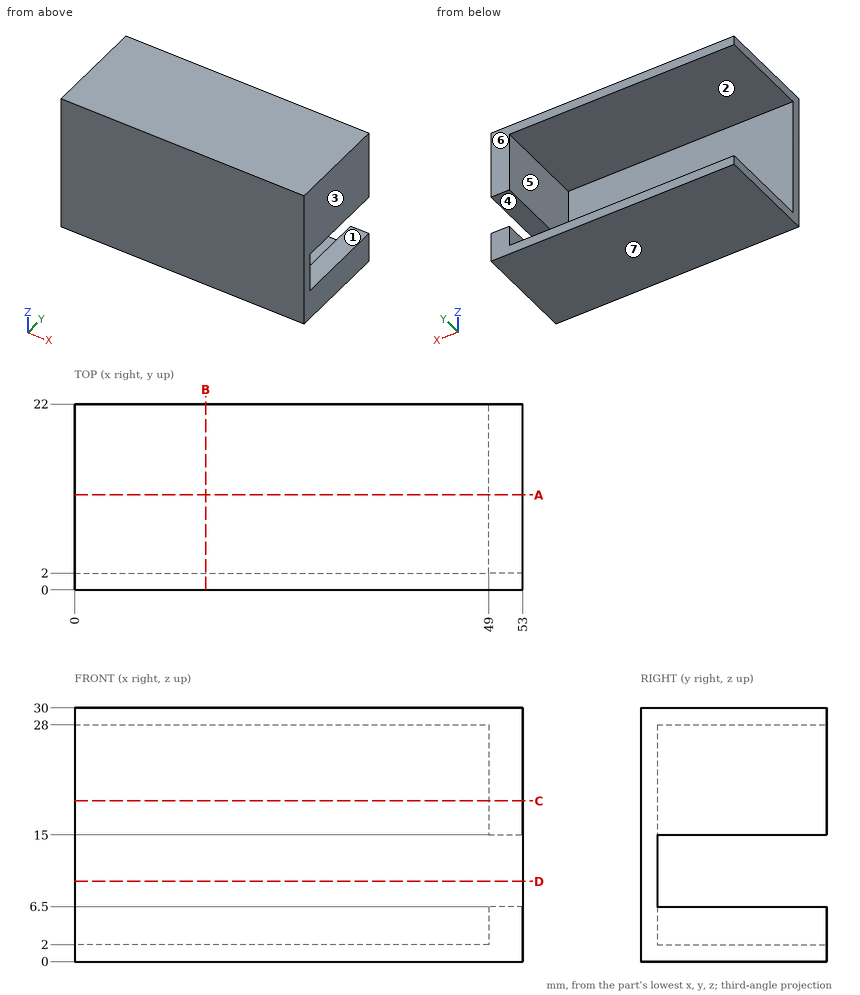
Here's the drawing with two shaded views (mm, measured from the low corner). I have some questions. A direction names the side the tool comes from. Give positions to 0.01 mm unless a question says otherwise; leave off trailing zeros. Loops run counter-clockwise (first coordinate to the right, second up) from the corner with the lowest first, then second, coordinate; pieces in that order, holes last. Notation, with made-up numbers: (61, 10) - (107, 10) arc R10 cw to (107, 14) - close; hole circle Ø10 at (1.5, 63). An arc over 180 degrees is marked (long way). Answer in a Markdown table with one row per item. Add a question column.
Q1. For pin 1 (3.5 mm diameter, centred on y = 16, z = 5, fed in from -X); pin 2 (8 mm diameter, centred on x = 15.5, z = 14.5, fed in from +Y), each with a flat end and sliding along its axis, tell me the tip position at first contact or that it passes through.
Q2. If we section it at D-D (z = 9.5): List the corners of the cut face in (x, y) for me, plus the area to 3 significant figures.
Q3. We'd pull the mould along Z, two halves only. Please class the marked faces 4, 5, 6 and 7: +Z half, -Z half, draft (parallel to the pull), parting line (faces both ways), or undercut.
Q4. If we section it at B-B (x = 15.5): List the corners of the cut face in (y, z) for me.
Q5. Please list where these lines run through material, in increasing order: L1, parallel to Z at x = 42, y = 9.25; L2, parallel to Y at x = 45, z = 12.5; L3, parallel to X at y = 6.75, z = 16.75. Write a range as from..to.
Q6. If we section it at C-C (z = 19): List the corners of the cut face in (x, y) for me.
Q7. If we section it at A-A (y = 11.25): List the corners of the cut face in (x, z) for me.
Q8. Which directions (+Z, -Z, +X, -X, +Y, -Y) give clear straight access to the entire face, cutting with the end or side of a thin tool? Please do the marked faces 1, 2 and 3.
The answers:
| question | item | result |
|---|---|---|
| 1 | pin 1 | stops at x = 49 |
| 1 | pin 2 | stops at y = 2 |
| 2 | outline | (0, 0) - (53, 0) - (53, 2) - (0, 2) - close |
| 2 | area | 106 mm^2 |
| 3 | face 4 | undercut |
| 3 | face 5 | undercut |
| 3 | face 6 | draft |
| 3 | face 7 | -Z half |
| 4 | outline | (0, 0) - (22, 0) - (22, 2) - (2, 2) - (2, 28) - (22, 28) - (22, 30) - (0, 30) - close |
| 5 | L1 | z = 0..2, 28..30 |
| 5 | L2 | y = 0..2 |
| 5 | L3 | x = 49..53 |
| 6 | outline | (0, 0) - (53, 0) - (53, 22) - (49, 22) - (49, 2) - (0, 2) - close |
| 7 | outline | (0, 0) - (53, 0) - (53, 6.5) - (49, 6.5) - (49, 2) - (0, 2) - close; (0, 28) - (49, 28) - (49, 15) - (53, 15) - (53, 30) - (0, 30) - close |
| 8 | face 1 | +X, -X, +Y |
| 8 | face 2 | -X, +Y |
| 8 | face 3 | +Z, -Z, +X, +Y, -Y |
